The model under review builds one solid part; all positions refer to its coordinate system, in mm. Coordinates: 2 decimals unless noted, no trailing zeros. Loops run counter-clockwise (first coordinate to the right, second up) from the corner with the lowest first, then second, coordinate; pieces in that order, holes last. Notation, with made-up numbers: (87, 4.25) - (99, 4.25) arc R25 cw to (99, 36.25) - close; hole circle Ø8 at (70.5, 41). An arc over 180 degrees is marked (long way). One line per item, written item: value. Start each with the question number.
1. To check wall thickness, follow line 1 (X direction, y = 1.75, z = 2.5); line 2 (Y direction, x = 3.25, z = 10) (3 decimals); line 3 (Z direction, x = -2, y = 5) (3 decimals). State the ranges of each line that lie inside material, in increasing order.
2. Insertion check: P1, Ø1.4, axis at x = -3.5, y = 7, coming from the +Z side (3 decimals); P2, Ø5, axis at y = -2.5, z = 4, coming from the -X side; P3, Ø1.4, axis at y = -3.18, z = 4.76, coming from the -X side; P4, Ø5, axis at y = -1, z = 6, coming from the +X side. Each pin has a flat end and moves straight along its axis. Give the tip position at first contact, or say it passes through.
3. We need section A-A, the plane z = 4. Give the boundary of the cut face in (x, y) (3 decimals).
4. We need section B-B, the plane x = 0.5. Count the separate pieces of the cut face and the enclosed holes in it, then the cut area to 3 significant figures.
5. We need section D-D, the plane z = 7.5. Give the boundary of the cut face in (x, y) (3 decimals), then the cut area to 3 significant figures.
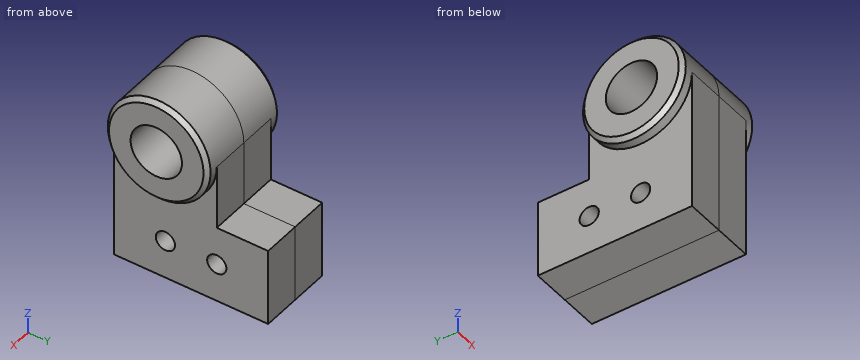
from build123d import *

# Parameters (mm, degrees)
F0_W     = 19.05
F0_H     = 9.525
F1_DEPTH = 4.699
F2_R     = 3.175
F3_DEPTH = 4.699
F4_R     = 1.190625
F5_DEPTH = 4.7
F6_R     = 6.35
F6_R_2   = 3.175
F7_DEPTH = 1.5875
F9_SIZE  = 0.508


with BuildPart() as f1:
    # F0 (on Right) → F1 (new body)
    with BuildSketch(Plane.YZ):
        with Locations((0, 4.7625)):
            Rectangle(F0_W, F0_H)
    extrude(amount=F1_DEPTH)

    # F2 (on Right) → F3 (join)
    with BuildSketch(Plane.YZ):
        with BuildLine():
            ThreePointArc((-9.525, 17.4625), (-3.175, 11.1125), (3.175, 17.4625))
            ThreePointArc((3.175, 17.4625), (-3.175, 23.8125), (-9.525, 17.4625))
        make_face()
        with Locations((-3.175, 17.4625)):
            Circle(F2_R, mode=Mode.SUBTRACT)
        with BuildLine():
            Line((3.175, 0), (3.175, 17.4625))
            ThreePointArc((3.175, 17.4625), (-3.175, 11.1125), (-9.525, 17.4625))
            Line((-9.525, 17.4625), (-9.525, 0))
            Line((-9.525, 0), (3.175, 0))
        make_face()
    extrude(amount=F3_DEPTH)

    # F4 (on face) → F5 (cut, through all)
    with BuildSketch(Plane.YZ.offset(4.699)):
        with Locations((-3.175, 4.7625)):
            Circle(F4_R)
        with Locations((3.175, 4.7625)):
            Circle(F4_R)
    extrude(amount=-F5_DEPTH, mode=Mode.SUBTRACT)

    # F6 (on face) → F7 (join)
    with BuildSketch(Plane.YZ.offset(4.699)):
        with Locations((-3.175, 17.4625)):
            Circle(F6_R)
        with Locations((-3.175, 17.4625)):
            Circle(F6_R_2, mode=Mode.SUBTRACT)
    extrude(amount=F7_DEPTH)

    # F8: F1 across plane


with BuildPart() as f1_1:
    add(f1.part)
    add(f1.part.mirror(Plane.YZ))

    # F9
    f9_edges = [f1_1.edges().sort_by_distance(p)[0] for p in [
        (6.2865, -9.525, 17.4625),
        (-6.2865, -9.525, 17.4625),
    ]]
    chamfer(f9_edges, length=F9_SIZE)


solid = f1_1.part
Findings below:
1. line 1: -4.7 to 4.7
1. line 2: -9.525 to 3.175
1. line 3: 0 to 9.525
2. P1: z = 9.525
2. P2: x = -4.7
2. P3: through
2. P4: x = 4.7
3. outline: (-4.699, -9.525) - (4.699, -9.525) - (4.699, -4.089) - (-4.699, -4.089) - close; (-4.699, -2.261) - (4.699, -2.261) - (4.699, 2.261) - (-4.699, 2.261) - close; (-4.699, 4.089) - (4.699, 4.089) - (4.699, 9.525) - (-4.699, 9.525) - close
4. separate pieces: 1
4. enclosed holes: 3
4. area: 305 mm2
5. outline: (-4.699, -9.525) - (4.699, -9.525) - (4.699, 9.525) - (-4.699, 9.525) - close
5. area: 179 mm2
